from build123d import *

# Parameters (mm, degrees)
SKETCH1_W            = 125
SKETCH1_H            = 100
BOSS_EXTRUDE1_DEPTH  = 2
CUT_EXTRUDE1_DEPTH   = 3
LPATTERN1_COUNT      = 6
LPATTERN1_PITCH      = 10
LPATTERN1_COUNT_DIR2 = 3
LPATTERN1_PITCH_DIR2 = 32.5
SKETCH3_R            = 2
CUT_EXTRUDE2_DEPTH   = 3
LPATTERN2_COUNT      = 6
LPATTERN2_PITCH      = 10
LPATTERN2_COUNT_DIR2 = 2
LPATTERN2_PITCH_DIR2 = 109.5
SKETCH4_R            = 2.5
CUT_EXTRUDE3_DEPTH   = 20
LPATTERN3_COUNT      = 5
LPATTERN3_PITCH      = 23.4
LPATTERN3_COUNT_DIR2 = 3
LPATTERN3_PITCH_DIR2 = 79.5


with BuildPart() as part:
    # Sketch1 → Boss-Extrude1 (new body)
    with BuildSketch(Plane(origin=(0, 0, 0), x_dir=(1, 0, 0), z_dir=(0, 1, 0))):
        Rectangle(SKETCH1_W, SKETCH1_H)
    extrude(amount=BOSS_EXTRUDE1_DEPTH)

    # Sketch2 → Cut-Extrude1 (cut, through all)
    with BuildSketch(Plane(origin=(0, 2, 0), x_dir=(1, 0, 0), z_dir=(0, 1, 0))):
        with BuildLine():
            Line((-43.604271847, 25.047104991), (-20.48386724, 25.047104991))
            ThreePointArc((-20.48386724, 25.047104991), (-18.658572139, 23.22180989), (-20.48386724, 21.39651479))
            Line((-20.48386724, 21.39651479), (-43.604271847, 21.39651479))
            ThreePointArc((-43.604271847, 21.39651479), (-45.429566947, 23.22180989), (-43.604271847, 25.047104991))
        make_face()
    cut_extrude1 = extrude(amount=-CUT_EXTRUDE1_DEPTH, mode=Mode.SUBTRACT)

    # LPattern1: Cut-Extrude1 6 × 3
    with Locations(*[(j * LPATTERN1_PITCH_DIR2, 0, i * LPATTERN1_PITCH) for i in range(LPATTERN1_COUNT) for j in range(LPATTERN1_COUNT_DIR2) if (i, j) != (0, 0)]):
        add(cut_extrude1, mode=Mode.SUBTRACT)

    # Sketch3 → Cut-Extrude2 (cut, through all)
    with BuildSketch(Plane(origin=(0, 2, 0), x_dir=(1, 0, 0), z_dir=(0, 1, 0))):
        with Locations((-54.55604245, 23.424620457)):
            Circle(SKETCH3_R)
    cut_extrude2 = extrude(amount=-CUT_EXTRUDE2_DEPTH, mode=Mode.SUBTRACT)

    # LPattern2: Cut-Extrude2 6 × 2
    with Locations(*[(j * LPATTERN2_PITCH_DIR2, 0, i * LPATTERN2_PITCH) for i in range(LPATTERN2_COUNT) for j in range(LPATTERN2_COUNT_DIR2) if (i, j) != (0, 0)]):
        add(cut_extrude2, mode=Mode.SUBTRACT)

    # Sketch4 → Cut-Extrude3 (cut)
    with BuildSketch(Plane(origin=(0, 2, 0), x_dir=(1, 0, 0), z_dir=(0, 1, 0))):
        with Locations((-46.240809214, 38.838223529)):
            Circle(SKETCH4_R)
    cut_extrude3 = extrude(amount=-CUT_EXTRUDE3_DEPTH, mode=Mode.SUBTRACT)

    # LPattern3: Cut-Extrude3 5 × 3
    with Locations(*[(i * LPATTERN3_PITCH, 0, j * LPATTERN3_PITCH_DIR2) for i in range(LPATTERN3_COUNT) for j in range(LPATTERN3_COUNT_DIR2) if (i, j) != (0, 0)]):
        add(cut_extrude3, mode=Mode.SUBTRACT)


solid = part.part
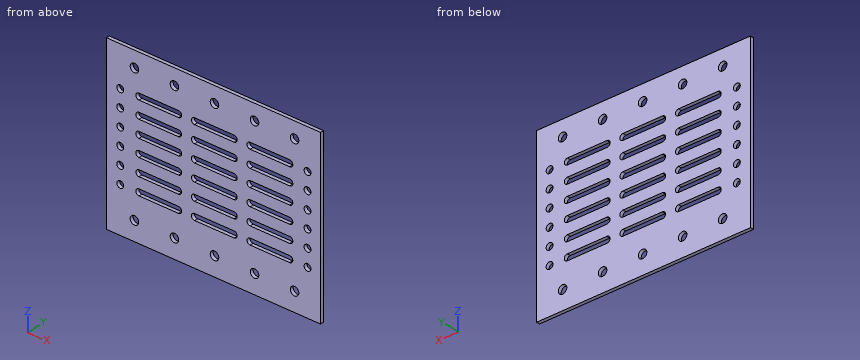
Can you work these out from the model? Positions are in its coordinate system, mm. Coordinates: 2 decimals unless noted, no trailing zeros. Loops run counter-clockwise (first coordinate to the right, second up) from the corner with the lowest first, then second, coordinate; pieces in that order, holes last. Notation, with made-up numbers: (-2, 26.5) - (49, 26.5) arc R29 ccw to (49, 58.5) - close; hole circle Ø1 at (20, 83.25). An arc over 180 degrees is marked (long way). Answer as a JSON object with one key per item and string values. Group by question number.
Item 1: If we section it at A-A (x = -34.5): List the corners of the cut face in (y, z) for me.
Item 2: If we section it at B-B (y = 1.65): State how many separate pieces and enclosed holes the cut face has, plus the area to 3 significant figures.
Item 3: For pin 1 (3 mm diameter, centred on x = 54.94, z = -23.42, fed in from -Y), with a flat end and sliding along its axis, tell me the tip position at first contact or that it passes through.
Item 4: If I drill on L1, parallel to X at y = 1.65, z = -22; L2, parallel to X at y = 0.3, z = 7; L3, parallel to Z at x = 46.5, y = 1.8, over which ranges is the centre line in solid material (lowest first)? Write a range as from..to.
Returned:
{
 "1": {"outline": "(0, -50) - (2, -50) - (2, -25.05) - (0, -25.05) - close; (0, -21.4) - (2, -21.4) - (2, -15.05) - (0, -15.05) - close; (0, -11.4) - (2, -11.4) - (2, -5.05) - (0, -5.05) - close; (0, -1.4) - (2, -1.4) - (2, 4.95) - (0, 4.95) - close; (0, 8.6) - (2, 8.6) - (2, 14.95) - (0, 14.95) - close; (0, 18.6) - (2, 18.6) - (2, 24.95) - (0, 24.95) - close; (0, 28.6) - (2, 28.6) - (2, 50) - (0, 50) - close"},
 "2": {"separate pieces": "1", "enclosed holes": "40", "area": "10,400 mm²"},
 "3": {"pin 1": "passes through"},
 "4": {"L1": "x = -62.5..-55.96, -53.15..-44.96, -19.13..-12.46, 13.37..20.04, 45.87..53.54, 56.35..62.5", "L2": "x = -62.5..-56.51, -52.6..-45.42, -18.67..-12.92, 13.83..19.58, 46.33..52.99, 56.9..62.5", "L3": "z = -50..-41.19, -36.49..38.31, 43.01..50"}
}
